Geometry: see drawing. Coordinates: mm, zero at the bounding-box minimum. A direction names the side the tool comes from. Give positions to 0.01 mm unless a question says otherwise; leave off trailing zeros. Order: outer loops, then holes, each group sorted by start corner. A loop starts at its lowest first (then second) coordinate and runs counter-clockwise, first axis right, second up. Notation, with made-up numbers: (-11, -23) -> (40, -23) arc R22 ccw to (40, -9) -> close; hole circle Ø11 at (-22.5, 17.25). An arc over 180 degrees is marked (long way). One line per item, written item: value. Start each with the question number.
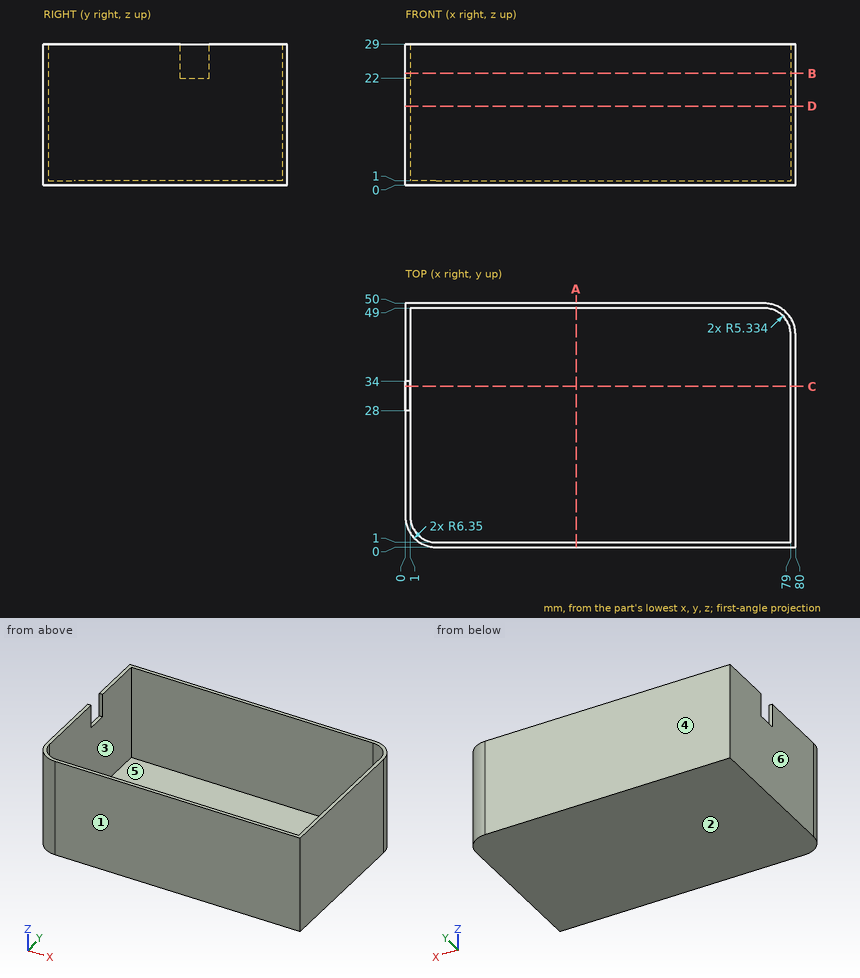
1. Cut plane C-C, the plane y = 33. Return loops of the section in (x, z).
2. Cut plane D-D, the plane z = 16.25. Return loops of the section in (x, y), then the cut area to 3 significant figures.
3. Pin query (flat end, axial travel): P1, Ø0.5, axis at x = 0.5, y = 32, coming from the +Z side; P2, Ø8, axis at x = 40, y = 23.5, coming from the +Z side; P3, Ø0.8, axis at x = 0.5, z = 24.5, coming from the -Y side. Return the tip coordinate at first contact, or that it passes through.
4. Access query for the marked faces 5 and 6. Directions: +Z, -Z, +X, -X, +Y, -Y. A direction counts if a zero-diameter tool reaches every point of the face in a straight line with its end or side. Return the directions, or none.
5. Material intervals for L1, parallel to Y at x = 45.5, z = 7.25; L2, parallel to X at y = 39, z = 4.5; L3, parallel to X at y = 30, z = 26, sorted ascending. Write a range as [from, to].
6. Cut plane A-A, the plane x = 35. Return loops of the section in (y, z), then the cut area to 3 significant figures.
7. Cut plane B-B, the plane z = 23. Return loops of the section in (x, y).
8. Draft query along Y for the marked faces 1, 2, 3 and 4. Return one class per face: pulls with the +Y half, pulls with the -Y half, needs draft (parallel to the pull), parting line crosses it, or undercut.
Answers follow:
1. outline: (0, 0) -> (80, 0) -> (80, 29) -> (79, 29) -> (79, 1) -> (1, 1) -> (1, 22) -> (0, 22) -> close
2. outline: (0, 6.35) arc R6.35 ccw to (6.35, 0) -> (80, 0) -> (80, 43.65) arc R6.35 ccw to (73.65, 50) -> (0, 50) -> close; hole (1, 6.33) arc R5.33 ccw to (6.33, 1) -> (79, 1) -> (79, 43.67) arc R5.33 ccw to (73.67, 49) -> (1, 49) -> close
2. area: 251 mm²
3. P1: stops at z = 22
3. P2: stops at z = 1
3. P3: stops at y = 3.09
4. face 5: +Z
4. face 6: +Z, -Z, -X, +Y, -Y
5. L1: y = [0, 1], [49, 50]
5. L2: x = [0, 1], [79, 80]
5. L3: x = [79, 80]
6. outline: (0, 0) -> (50, 0) -> (50, 29) -> (49, 29) -> (49, 1) -> (1, 1) -> (1, 29) -> (0, 29) -> close
6. area: 106 mm²
7. outline: (0, 6.35) arc R6.35 ccw to (6.35, 0) -> (80, 0) -> (80, 43.65) arc R6.35 ccw to (73.65, 50) -> (0, 50) -> (0, 34) -> (1, 34) -> (1, 49) -> (73.67, 49) arc R5.33 cw to (79, 43.67) -> (79, 1) -> (6.33, 1) arc R5.33 cw to (1, 6.33) -> (1, 28) -> (0, 28) -> close
8. face 1: pulls with the -Y half
8. face 2: needs draft
8. face 3: undercut
8. face 4: pulls with the +Y half
